Autodesk Fusion 360 part; units mm, degrees
sketch "Sketch1" plane through (0, 0, 0) normal (0, 0, 1) x (1, 0, 0)
  line L0 (0, 0) -> (50, 0)
  line L1 (50, 0) -> (50, -55)
  line L2 (50, -55) -> (0, -55)
  line L3 (0, -55) -> (0, 0)
  line L4 (7, -12.5) -> (37, -12.5)
  line L5 (37, -12.5) -> (37, -42.5)
  line L6 (37, -42.5) -> (7, -42.5)
  line L7 (7, -42.5) -> (7, -12.5)
  dimension "d7" = 50
  dimension "d8" = 55
  dimension "d15" = 30
  dimension "d16" = 30
  dimension "d17" = 7
  dimension "d18" = 12.5
extrude "Extrude1" add sketch "Sketch1" along normal blind 5 contours L0 L1 L2 L3 | L4 L5 L6 L7
extrude "Extrude2" cut sketch "Sketch1" along normal blind 100 contours L4 L5 L6 L7
equation "perfboard_length = 35 mm"
equation "perfboard_width = 30 mm"
equation "width = perfboard_length + 2 * screw_radius * 2"
equation "length = perfboard_width + 2 * screw_radius * 2"
equation "height = 5 mm"
equation "d7 = length"
equation "d8 = width"
equation "d9 = height"
equation "middle_gap_width = 30 mm"
equation "middle_gap_length = length - 2 * screw_radius * 2"
equation "middle_gap_small_distance = 7 mm"
equation "middle_gap_big_distance = ( width - middle_gap_width ) / 2"
equation "d15 = middle_gap_length"
equation "d16 = middle_gap_width"
equation "d17 = middle_gap_small_distance"
equation "d18 = middle_gap_big_distance"
equation "extra = 100 mm"
equation "d20 = extra"
equation "screw_radius = 5 mm"
CAD build for the part. Positions are in the model's coordinates, mm. A direction names the side the tool comes from. Coordinates: 2 decimals unless noted, no trailing zeros. Order: outer loops, then holes, each group sorted by start corner. A loop starts at its lowest first (then second) coordinate and runs counter-clockwise, first axis right, second up. Notation, with made-up numbers: (16, 11) - (68, 11) arc R36 cw to (68, 47) - close; hole circle Ø3 at (8.25, -7). An arc over 180 degrees is marked (long way). Answer in a Markdown table with one row per item.
1. Slice it at B-B, the plane z = 3.1. List the corners of the cut face in (x, y).
Answer:
| item | result |
|---|---|
| outline | (0, -55) - (50, -55) - (50, 0) - (0, 0) - close; hole (7, -42.5) - (37, -42.5) - (37, -12.5) - (7, -12.5) - close |
2. Drill centre lines: L1, parallel to Y at x = 10.5, z = 3.35; L2, parallel to X at y = -25.5, z = 2.05. Where is each one in solid material? Low to high. Write a range as from..to.
Answer:
| item | result |
|---|---|
| L1 | -55..-42.5, -12.5..0 |
| L2 | 0..7, 37..50 |
3. 3-axis set-ups, long thin cutter, end or side, ignore diameter. For faces 1 (the face through (25, -55, 2)), 2 (the face through (7, -28, 2)): which of +Z, -Z, +X, -X, +Y, -Y reach the whole face in a straight line?
Answer:
| item | result |
|---|---|
| face 1 | +Z, -Z, +X, -X, -Y |
| face 2 | +Z, -Z |
4. Pull direction X, two halves, no side cores. Call faces 3 (the face through (25, 0, 2)), 4 (the face through (37, -27, 2)), 5 (the face through (50, -27, 2)): +X half, -X half, draft (parallel to the pull), parting line (faces both ways), or undercut.
Answer:
| item | result |
|---|---|
| face 3 | draft |
| face 4 | undercut |
| face 5 | +X half |
5. Slice it at C-C, the plane x = 26. List the corners of the cut face in (y, z), then the cut area to 3 significant figures.
Answer:
| item | result |
|---|---|
| outline | (-55, 0) - (-42.5, 0) - (-42.5, 5) - (-55, 5) - close; (-12.5, 0) - (0, 0) - (0, 5) - (-12.5, 5) - close |
| area | 125 mm² |
6. Slice it at A-A, the plane y = -30.5. List the corners of the cut face in (x, z).
Answer:
| item | result |
|---|---|
| outline | (0, 0) - (7, 0) - (7, 5) - (0, 5) - close; (37, 0) - (50, 0) - (50, 5) - (37, 5) - close |
